```python
from build123d import *

# Parameters (mm, degrees)
SKETCH1_R           = 1.5
BOSS_EXTRUDE1_DEPTH = 4
SKETCH2_W           = 3
SKETCH2_H           = 51.803847578
SKETCH2_W_2         = 66.803847578
SKETCH2_H_2         = 3
CUT_EXTRUDE1_DEPTH  = 3


with BuildPart() as part:
    # Sketch1 → Boss-Extrude1 (new body)
    with BuildSketch(Plane(origin=(0, 0, 0), x_dir=(1, 0, 0), z_dir=(0, 1, 0))):
        with BuildLine():
            Line((-33.401923789, 30), (33.401923789, 30))
            ThreePointArc((33.401923789, 30), (38.121320344, 30.621320344), (37.5, 25.901923789))
            Line((37.5, 25.901923789), (37.5, -25.901923789))
            ThreePointArc((37.5, -25.901923789), (38.121320344, -30.621320344), (33.401923789, -30))
            Line((33.401923789, -30), (-33.401923789, -30))
            ThreePointArc((-33.401923789, -30), (-38.121320344, -30.621320344), (-37.5, -25.901923789))
            Line((-37.5, -25.901923789), (-37.5, 25.901923789))
            ThreePointArc((-37.5, 25.901923789), (-38.121320344, 30.621320344), (-33.401923789, 30))
        make_face()
        with Locations(Location((36, 28.5, 0), (0, 0, 270))):
            Circle(SKETCH1_R, mode=Mode.SUBTRACT)
        with Locations(Location((36, -28.5, 0), (0, 0, 270))):
            Circle(SKETCH1_R, mode=Mode.SUBTRACT)
        with Locations(Location((-36, -28.5, 0), (0, 0, 270))):
            Circle(SKETCH1_R, mode=Mode.SUBTRACT)
        with Locations(Location((-36, 28.5, 0), (0, 0, 270))):
            Circle(SKETCH1_R, mode=Mode.SUBTRACT)
        with BuildLine():
            Line((-33.401923789, 27), (33.401923789, 27))
            ThreePointArc((33.401923789, 27), (33.878679656, 26.378679656), (34.5, 25.901923789))
            Line((34.5, 25.901923789), (34.5, -25.901923789))
            ThreePointArc((34.5, -25.901923789), (33.878679656, -26.378679656), (33.401923789, -27))
            Line((33.401923789, -27), (-33.401923789, -27))
            ThreePointArc((-33.401923789, -27), (-33.878679656, -26.378679656), (-34.5, -25.901923789))
            Line((-34.5, -25.901923789), (-34.5, 25.901923789))
            ThreePointArc((-34.5, 25.901923789), (-33.878679656, 26.378679656), (-33.401923789, 27))
        make_face(mode=Mode.SUBTRACT)
    extrude(amount=BOSS_EXTRUDE1_DEPTH)

    # Sketch2 → Cut-Extrude1 (cut)
    with BuildSketch(Plane(origin=(0, 4, 0), x_dir=(1, 0, 0), z_dir=(0, 1, 0))):
        with Locations((-36, 0)):
            Rectangle(SKETCH2_W, SKETCH2_H)
        with Locations((0, -28.5)):
            Rectangle(SKETCH2_W_2, SKETCH2_H_2)
        with Locations((36, 0)):
            Rectangle(SKETCH2_W, SKETCH2_H)
        with Locations((0, 28.5)):
            Rectangle(SKETCH2_W_2, SKETCH2_H_2)
    extrude(amount=-CUT_EXTRUDE1_DEPTH, mode=Mode.SUBTRACT)


solid = part.part
```
Verification items for the finished model (mm, model axes). A direction names the side the tool comes from. Coordinates: 2 decimals unless noted, no trailing zeros. Loops run counter-clockwise (first coordinate to the right, second up) from the corner with the lowest first, then second, coordinate; pieces in that order, holes last. Notation, with made-up numbers: (85, -38) - (98, -38) arc R16 cw to (98, -13) - close; hole circle Ø8 at (14, 48). An arc over 180 degrees is marked (long way). Return JSON: item names as keys, results as strings.
1. Mould release check, pull along Z, two halves, no side actions. Record for faces 4 (the flat face through (33.402, 3, 29)), 5 (the flat face through (36, 1, 0)), 6 (the cylindrical face through (-38.175, 1.972, -30.566)): +Z half, -Z half, draft (parallel to the pull), parting line (faces both ways), or undercut.
Established:
{"face 4": "draft", "face 5": "undercut", "face 6": "undercut"}
2. Go/stop test with flat-tipped pins: pin 1 (0.8 mm diameter, centred on y = 0.5, z = 12, fed in from -X); pin 2 (1.5 mm diameter, centred on x = -3.5, z = 28, fed in from +Y); pin 3 (0.5 mm diameter, centred on x = -8, y = 0.5, fed in from -Z). Record where each tip stops, or that it passes through.
Established:
{"pin 1": "stops at x = -37.5", "pin 2": "stops at y = 1", "pin 3": "stops at z = -30"}
3. Section check D-D, the plane z = 17.5. Record the boundary of the cut face in (x, y), then the cut area to 3 significant figures.
Established:
{"outline": "(-37.5, 0) - (-34.5, 0) - (-34.5, 1) - (-37.5, 1) - close; (34.5, 0) - (37.5, 0) - (37.5, 1) - (34.5, 1) - close", "area": "6.00 mm2"}
4. Thickness scan on L1, parallel to X at y = 3.2, z = 28.5; L2, parallel to X at y = 1.5, z = -27.5; L3, parallel to Z at x = 12, y = 0.7. Record the ranges inside material, lowest first.
Established:
{"L1": "x = -39 to -37.5, -34.5 to -33.4, 33.4 to 34.5, 37.5 to 39", "L2": "x = -38.83 to -37.12, -34.88 to -33.4, 33.4 to 34.88, 37.12 to 38.83", "L3": "z = -30 to -27, 27 to 30"}
5. Section check C-C, the plane x = 21. Record the boundary of the cut face in (y, z), then the cut area to 3 significant figures.
Established:
{"outline": "(0, -30) - (1, -30) - (1, -27) - (0, -27) - close; (0, 27) - (1, 27) - (1, 30) - (0, 30) - close", "area": "6.00 mm2"}
6. Section check B-B, the plane y = 1.95. Record the boundary of the cut face in (x, z), then the cut area to 3 significant figures.
Established:
{"outline": "(-37.5, -25.9) arc R3 ccw (long way) to (-33.4, -30) - (-33.4, -27) arc R3 ccw to (-34.5, -25.9) - close; (-37.5, 25.9) - (-34.5, 25.9) arc R3 ccw to (-33.4, 27) - (-33.4, 30) arc R3 ccw (long way) to start; (33.4, -30) arc R3 ccw (long way) to (37.5, -25.9) - (34.5, -25.9) arc R3 ccw to (33.4, -27) - close; (33.4, 27) arc R3 ccw to (34.5, 25.9) - (37.5, 25.9) arc R3 ccw (long way) to (33.4, 30) - close; hole circle Ø3 at (-36, -28.5); hole circle Ø3 at (-36, 28.5); hole circle Ø3 at (36, -28.5); hole circle Ø3 at (36, 28.5)", "area": "78.3 mm2"}
7. Tool access check on faces 1 (the flat face through (-36, 1, 0)), 2 (the flat face through (-37, 4, -30)), 3 (the flat face through (0, 1, 28)). Record the directions out of +Z, -Z, +X, -X, +Y, -Y that give a thin tool (end or side, any length) a straight path to the whole face; none if there is none.
Established:
{"face 1": "+X, -X, +Y", "face 2": "+Z, -Z, +X, -X, +Y", "face 3": "+Z, -Z, +Y"}
8. Section check A-A, the plane z = -28.5. Record the boundary of the cut face in (x, y), then the cut area to 3 significant figures.
Established:
{"outline": "(-39, 0) - (-37.5, 0) - (-37.5, 4) - (-39, 4) - close; (-34.5, 0) - (34.5, 0) - (34.5, 4) - (33.4, 4) - (33.4, 1) - (-33.4, 1) - (-33.4, 4) - (-34.5, 4) - close; (37.5, 0) - (39, 0) - (39, 4) - (37.5, 4) - close", "area": "87.6 mm2"}
